Answer from the drawing. Dimensions are ordinates in mm from the lowest x, y and z of the part. A direction names the side the tool comes from. Round coordinates to 2 decimals unless told otherwise and drop trailing zeros. Order: outer loops, then holes, each group sorted by start corner. A loop starts at its lowest first (then second) coordinate and runs counter-clockwise, first axis right, second up. Notation, with made-up numbers: (-6, 16.25) -> (10, 16.25) arc R21 cw to (10, 52.25) -> close; hole circle Ø9 at (-26.5, 12.25). An arc over 180 degrees is marked (long way). Use a Markdown table: item, result. Add a question column.
Item 1: A cutting plane is placed at B-B, the plane z = 3.2. Determine the outline of the cut face in (x, y), plus the area to 3 significant figures.
Item 2: For a pull along X with two mould halves and no side action, classify the marked faces 4, 5 and 6 as +X half, -X half, draft (parallel to the pull), parting line (faces both ways), or undercut.
Item 3: A cutting plane is placed at C-C, the plane x = 18.25. Determine the outline of the cut face in (y, z) (1 decimal).
Item 4: A cutting plane is placed at A-A, the plane x = 12. Determine the outline of the cut face in (y, z).
Item 5: A tool of negligible diameter and unlimited length cuts with its end or side. For the marked faces 1, 2 and 3, from which of +Z, -Z, +X, -X, +Y, -Y can it reach the whole face along a straight path? Write none if from no direction.
Item 6: Flat-ended cylindrical pins translate along their axes: P1, Ø10, axis at x = 16.5, y = 19.5, coming from the +Z side; P2, Ø3, axis at x = 6, z = 1.5, coming from the +Y side (1 decimal); P3, Ø1.5, axis at y = 19.5, z = 2.5, coming from the +X side; P4, Ø3, axis at y = 19, z = 3.5, coming from the -X side. Find the tip coordinate at first contact, or state that the pin passes through.
Item 7: A cutting plane is placed at D-D, the plane y = 25.5. Determine the outline of the cut face in (x, z), plus the area to 3 significant figures.
Item 8: Find the intervals of material crossed by L1, parallel to Y at x = 12, z = 1.9; L2, parallel to X at y = 9, z = 2.95; L3, parallel to Y at x = 6, z = 4.5 (1 decimal), in increasing order. Write a range as [from, to].
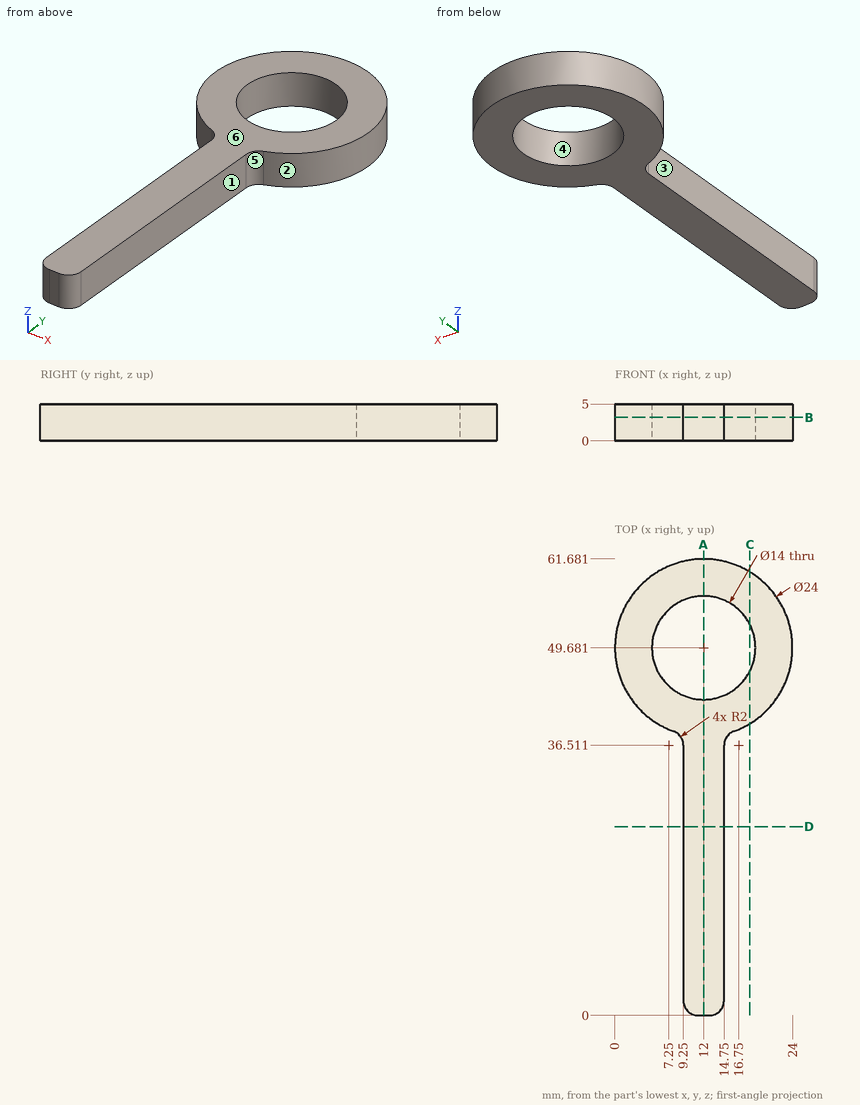
Reported:
| question | item | result |
|---|---|---|
| 1 | outline | (7.93, 38.39) arc R2 cw to (9.25, 36.51) -> (9.25, 2) arc R2 ccw to (11.25, 0) -> (12.75, 0) arc R2 ccw to (14.75, 2) -> (14.75, 36.51) arc R2 cw to (16.07, 38.39) arc R12 ccw (long way) to start; hole circle Ø14 at (12, 49.68) |
| 1 | area | 505 mm² |
| 2 | face 4 | undercut |
| 2 | face 5 | +X half |
| 2 | face 6 | draft |
| 3 | outline | (39.4, 0) -> (46.5, 0) -> (46.5, 5) -> (39.4, 5) -> close; (52.8, 0) -> (59.9, 0) -> (59.9, 5) -> (52.8, 5) -> close |
| 4 | outline | (0, 0) -> (42.68, 0) -> (42.68, 5) -> (0, 5) -> close; (56.68, 0) -> (61.68, 0) -> (61.68, 5) -> (56.68, 5) -> close |
| 5 | face 1 | +Z, -Z, +X, -Y |
| 5 | face 2 | +Z, -Z |
| 5 | face 3 | +Z, -Z, -X, -Y |
| 6 | P1 | z = 5 |
| 6 | P2 | y = 60.8 |
| 6 | P3 | x = 14.75 |
| 6 | P4 | x = 9.25 |
| 7 | outline | (9.25, 0) -> (14.75, 0) -> (14.75, 5) -> (9.25, 5) -> close |
| 7 | area | 27.5 mm² |
| 8 | L1 | [0, 42.68], [56.68, 61.68] |
| 8 | L2 | [9.25, 14.75] |
| 8 | L3 | [39.3, 46.1], [53.3, 60.1] |
